```python
from build123d import *

# Parameters (mm, degrees)
F2_ANGLE = 180


with BuildPart() as f2:
    # F1 (on Front) → F2 (revolve)
    with BuildSketch(Plane.XZ):
        Polygon((-68.0832503253, 1.2704479365), (-65.8827699508, 0), (-68.0832503253, -1.2704479365), (-67.590510429, -2.1238883528), (-65.6038210217, -0.9768590888), (-62.4301136979, -6.4738162454), (-59.2582268861, -11.9676853595), (-61.244893976, -13.1146881387), (-60.7503676631, -13.9712226825), (-58.5499524964, -12.7008123937), (-58.5499524964, -15.2283469215), (-57.5584731996, -15.2283469215), (-57.5584731996, -12.9530243576), (-51.217135042, -12.9530243576), (-44.862665236, -12.9530243576), (-44.862665236, -15.2283469215), (-43.8843175875, -15.2283469215), (-43.8843175875, -12.7008123937), (-41.6742515512, -13.9767946147), (-41.1808964662, -13.1190662144), (-43.1607244284, -11.9802929242), (-39.9959231548, -6.4780897113), (-36.8304619331, -0.9747391376), (-34.850633971, -2.1135124278), (-34.3620503103, -1.2640794445), (-36.5515001331, 0), (-34.3620503103, 1.2640794445), (-34.8630113186, 2.1323707922), (-36.8285001335, 0.9983813071), (-39.9917026714, 6.4810064009), (-43.1661904902, 11.9793805911), (-41.19939244, 13.1149119748), (-41.6910577545, 13.9670915487), (-43.8843175875, 12.7008123937), (-43.8843175875, 15.2525296435), (-44.861279428, 15.2523063589), (-44.861279428, 12.9604106769), (-51.217135042, 12.9604106769), (-57.5630575919, 12.9604106769), (-57.5630575919, 15.2494033683), (-58.5499524964, 15.2491778135), (-58.5499524964, 12.7008123937), (-60.7598529608, 13.9766990217), (-61.2508664965, 13.1247800337), (-59.2498548651, 11.9714734282), (-62.425474964, 6.4711380712), (-65.6057968908, 0.9626589096), (-67.5986398816, 2.1112574229), align=None)
        with BuildLine():
            ThreePointArc((-51.217135042, 12.7008123937), (-42.2363044718, 8.9808305702), (-38.5163226482, 0))
            ThreePointArc((-38.5163226482, 0), (-60.1979656121, -8.9808305702), (-51.217135042, 12.7008123937))
        make_face(mode=Mode.SUBTRACT)
    revolve(axis=Axis((0, 0, 0), (0, 0, 1)), revolution_arc=F2_ANGLE)


solid = f2.part
```
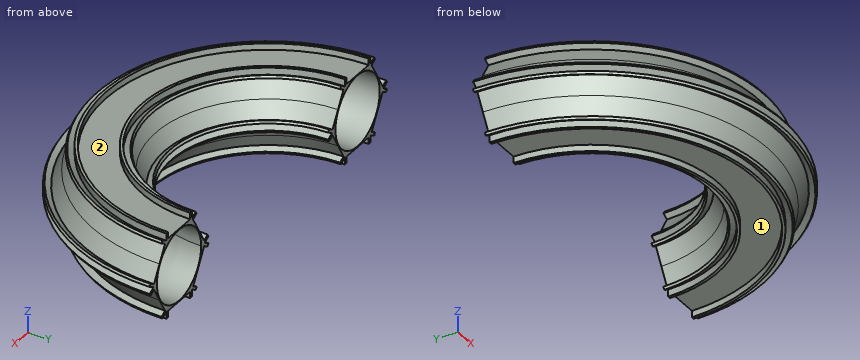
Work out the finished part from the listing and answer in its coordinate system (mm). Face numbers are marked on the shaded views. A direction names the side the tool comes from. Give positions to 0.01 mm unless a question says otherwise; leave off trailing zeros. Loops run counter-clockwise (first coordinate to the right, second up) from the corner with the lowest first, then second, coordinate; pieces in that order, holes last. Notation, with made-up numbers: (46, 78) -> (102, 78) arc R11 cw to (102, 94) -> close; hole circle Ø1 at (-23, 11.25). An arc over 180 degrees is marked (long way). Use CSV: the item, a comma, the result in double quotes.
1. The part is cut by section A-A (z = 10.5). Write down the section's boundary in (x, y), then the cut area to 3 significant figures.
Found:
outline,"(-60.1, 0) arc R60.1 ccw to (60.1, 0) -> (58.36, 0) arc R58.36 cw to (-58.36, 0) -> close; (-44.07, 0) arc R44.07 ccw to (44.07, 0) -> (42.31, 0) arc R42.31 cw to (-42.31, 0) -> close"
area,"562 mm^2"
2. A tool of negligible diameter and unlimited length cuts with its end or side. For the marked faces 1 and 2, from which of +Z, -Z, +X, -X, +Y, -Y can it reach the whole face along a straight path? Write none if from no direction.
Found:
face 1,"-Z"
face 2,"+Z"
3. Flat-ended cylindrical pins translate along their axes: pin 1 Ø3 at (x, z) = (-13, -3.5) entering from -Y; pin 2 Ø1.5 at (y, z) = (-21.5, -9) entering from -X; pin 3 Ø10 at (y, z) = (-39, -3.5) entering from +X; pin 4 Ø10 at (x, y) = (42, -61) entering from -Z. Find the tip coordinate at first contact, or state that the pin passes through.
Found:
pin 1,"y = -66.45"
pin 2,"x = -57.59"
pin 3,"x = 58.68"
pin 4,"through"
4. Straight lines are drawn through the part: line 1 (X direction, y = -28, z = 3.5); line 2 (X direction, y = -7, z = 6); line 3 (Z direction, x = 25.5, y = -34.5). For each, find the intervals that lie inside material, in ascending order.
Found:
line 1,"-57.71 to -56.91, -27.16 to -26.09, 26.09 to 27.16, 56.91 to 57.71"
line 2,"-62.31 to -62.02, -39.41 to -39.09, 39.09 to 39.41, 62.02 to 62.31"
line 3,"-13.27 to -12.13, -11.53 to -9.6, 9.6 to 11.52, 12.13 to 13.27"
5. The part is cut by section B-B (y = -14). State how many separate pieces and enclosed holes the cut face has, then the cut area to 3 significant figures.
Found:
separate pieces,"2"
enclosed holes,"2"
area,"212 mm^2"
